```python
from build123d import *

# Parameters (mm, degrees)
BOSS_EXTRUDE1_DEPTH = 15
BOSS_EXTRUDE2_DEPTH = 17.29


with BuildPart() as part:
    # Sketch2 → Boss-Extrude1 (new body)
    with BuildSketch(Plane(origin=(0, 0, 0), x_dir=(1, 0, 0), z_dir=(0, 1, 0))):
        Polygon((0, 0), (15, 0), (11.643601475, 4), (13.143601475, 4), (16.143601475, 4), (16.143601475, -1), (-1.143601475, -1), (-1.143601475, 4), (1.856398525, 4), (3.356398525, 4), align=None)
    extrude(amount=BOSS_EXTRUDE1_DEPTH)

    # Sketch5 → Boss-Extrude2 (add)
    with BuildSketch(Plane(origin=(16.143601475, 0, 0), x_dir=(0, 0, -1), z_dir=(1, 0, 0))):
        with BuildLine():
            Line((-1, 2.25), (-4.43, 2.25))
            ThreePointArc((-4.43, 2.25), (-8.432605401, 2.437913267), (-12.4, 3))
            Line((-12.4, 3), (-12.4, 0))
            Line((-12.4, 0), (-1, 0))
            Line((-1, 0), (-1, 2.25))
        make_face()
        with BuildLine():
            Line((-1, 12.75), (-4.43, 12.75))
            ThreePointArc((-4.43, 12.75), (-8.432605401, 12.562086733), (-12.4, 12))
            Line((-12.4, 12), (-12.4, 15))
            Line((-12.4, 15), (-1, 15))
            Line((-1, 15), (-1, 12.75))
        make_face()
    extrude(amount=-BOSS_EXTRUDE2_DEPTH)


solid = part.part
```
Work out the finished part from the listing and answer in its coordinate system (mm). A direction names the side the tool comes from. Give positions to 0.01 mm unless a question says otherwise; leave off trailing zeros. Order: outer loops, then holes, each group sorted by start corner. A loop starts at its lowest first (then second) coordinate and runs counter-clockwise, first axis right, second up. Notation, with made-up numbers: (8.5, 87.25) - (14.5, 87.25) arc R28 cw to (14.5, 124.25) - close; hole circle Ø4 at (67.5, 57.25). An arc over 180 degrees is marked (long way). One line per item, written item: value. Start each with the question number.
1. Section B-B, the plane x = 2.25 is taken. Write down the section's boundary in (y, z), then the cut area to 3 significant figures.
2. For a pull along Y with two mould halves and no side action, classify faces 4 (the face through (8, 0, 6)), 5 (the face through (8, 7, 1)), 6 (the face through (13.345, 7.395, -1.972)), 7 (the face through (7.62, 12.567, 8.377)) as released by +Y, released by -Y, zero draft, split by the parting line, or undercut.
3. Section A-A, the plane z = 3.75 is taken. Write down the section's boundary in (x, y).
4. Each of these flat-tipped pins is pushed along its axis until it touches: pin 1 Ø6 at (y, z) = (9.5, 8.5) entering from +X; pin 2 Ø6 at (x, y) = (11, 8) entering from +Z; pin 3 Ø4 at (y, z) = (5, -1.5) entering from -X. Where does it stop, or does it pass through?
5. Consider line 1 (Z direction, x = 5.25, y = 10); line 2 (Y direction, x = 15.25, z = 7); line 3 (Z direction, x = 7, y = 1.75). Determine where each line is inside the solid, lowest interval first.
6. Section D-D, the plane x = 10 is taken. Write down the section's boundary in (y, z).
7. Which of the six approach directions +Z, -Z, +X, -X, +Y, -Y give full straight-line access (tool end or side, diameter ignored) to faces 1 (the face through (8, 12.75, 3)), 2 (the face through (1, 7, -4)), 3 (the face through (7, 7, 0))?
Filled sheet:
1. outline: (0, -4) - (15, -4) - (15, -2.68) - (0, -2.68) - close; (0, 0) - (15, 0) - (15, 12.4) - (12, 12.4) arc R42.72 cw to (12.75, 4.43) - (12.75, 1) - (2.25, 1) - (2.25, 4.43) arc R42.72 cw to (3, 12.4) - (0, 12.4) - close
1. area: 90.0 mm²
2. face 4: released by -Y
2. face 5: undercut
2. face 6: zero draft
2. face 7: undercut
3. outline: (-1.15, 0) - (16.14, 0) - (16.14, 2.25) - (-1.15, 2.25) - close; (-1.15, 12.75) - (16.14, 12.75) - (16.14, 15) - (-1.15, 15) - close
4. pin 1: through
4. pin 2: z = 1
4. pin 3: x = -1.14
5. line 1: 0 to 1
5. line 2: 0 to 2.33, 12.67 to 15
5. line 3: 0 to 12.4
6. outline: (0, 0) - (15, 0) - (15, 12.4) - (12, 12.4) arc R42.72 cw to (12.75, 4.43) - (12.75, 1) - (2.25, 1) - (2.25, 4.43) arc R42.72 cw to (3, 12.4) - (0, 12.4) - close
7. face 1: +X, -X
7. face 2: -Z, +X, -X, +Y, -Y
7. face 3: +Y, -Y
